Work out the finished part from the listing and answer in its coordinate system (mm). A direction names the side the tool comes from. Round coordinates to 2 decimals unless told otherwise and drop trailing zeros. Order: outer loops, then holes, each group sorted by start corner. A loop starts at its lowest first (then second) coordinate and runs counter-clockwise, first axis right, second up. Notation, with made-up numbers: M -14.5,38 L 14.5,38 A6 cw 14.5,45 Z; hole C 73,19 d8. An arc over 180 degrees is marked long. Return JSON: item names as keys, results as strings.
from build123d import *

# Parameters (mm, degrees)
SKETCH2_W           = 508
SKETCH2_H           = 101.6
BOSS_EXTRUDE2_DEPTH = 965.2
SKETCH3_R           = 25.4
SKETCH3_W           = 25.4
SKETCH3_H           = 25.4
CUT_EXTRUDE1_DEPTH  = 50.8
FILLET1_R           = 203.2
FILLET2_R           = 203.2
FILLET4_R           = 43.18


with BuildPart() as part:
    # Sketch2 → Boss-Extrude2 (new body)
    with BuildSketch(Plane.XY):
        with Locations((254, 50.8)):
            Rectangle(SKETCH2_W, SKETCH2_H)
    extrude(amount=BOSS_EXTRUDE2_DEPTH)

    # Sketch3 → Cut-Extrude1 (cut)
    with BuildSketch(Plane(origin=(0, 0, 0), x_dir=(-1, 0, 0), z_dir=(0, -1, 0))):
        with Locations(Location((-88.9, -736.6, 0), (0, 0, 90))):
            Circle(SKETCH3_R)
        with Locations(Location((-419.1, -736.6, 0), (0, 0, 90))):
            Circle(SKETCH3_R)
        with Locations((-393.7, -228.6)):
            Rectangle(SKETCH3_W, SKETCH3_H)
        with Locations((-114.3, -228.6)):
            Rectangle(SKETCH3_W, SKETCH3_H)
    extrude(amount=-CUT_EXTRUDE1_DEPTH, mode=Mode.SUBTRACT)

    # Fillet1
    fillet1_edges = [part.edges().sort_by_distance(p)[0] for p in [
        (0, 50.8, 965.2),
    ]]
    fillet(fillet1_edges, radius=FILLET1_R)

    # Fillet2
    fillet2_edges = [part.edges().sort_by_distance(p)[0] for p in [
        (508, 50.8, 965.2),
    ]]
    fillet(fillet2_edges, radius=FILLET2_R)

    # Fillet4
    fillet4_edges = [part.edges().sort_by_distance(p)[0] for p in [
        (254, 101.6, 965.2),
        (0, 101.6, 381),
        (59.515902063, 101.6, 905.684097937),
        (508, 101.6, 381),
        (254, 101.6, 0),
        (448.484097937, 101.6, 905.684097937),
    ]]
    fillet(fillet4_edges, radius=FILLET4_R)


solid = part.part
Item 1: Which of the six approach directions +Z, -Z, +X, -X, +Y, -Y give full straight-line access (tool end or side, diameter ignored) to faces 4 (the flat face through (251, 101.6, 476)), 5 (the flat face through (101.6, 25, 229))?
Output:
{"face 4": "+Z, -Z, +X, -X, +Y", "face 5": "-Y"}
Item 2: Find section B-B (z = 736.6). Determine the outline of the cut face in (x, y).
Output:
{"outline": "M 0,0 L 63.5,0 L 63.5,50.8 L 114.3,50.8 L 114.3,0 L 393.7,0 L 393.7,50.8 L 444.5,50.8 L 444.5,0 L 508,0 L 508,58.42 A43.18 ccw 464.82,101.6 L 43.18,101.6 A43.18 ccw 0,58.42 Z"}
Item 3: Consider line 1 along X through (y, z) = (18.5, 736.6); line 2 along Y through (x, z) = (398, 227.5); line 3 along Y through (x, z) = (467.5, 134.5). Determine where each line is inside the solid, lowest interval first. Write a range as [from, to].
Output:
{"line 1": "x = [0, 63.5], [114.3, 393.7], [444.5, 508]", "line 2": "y = [50.8, 101.6]", "line 3": "y = [0, 101.52]"}
Item 4: Find section C-C (z = 60.5). Determine the outline of the cut face in (x, y).
Output:
{"outline": "M 0,0 L 508,0 L 508,58.42 A43.18 ccw 464.82,101.6 L 43.18,101.6 A43.18 ccw 0,58.42 Z"}
Item 5: Each of these flat-tipped pins is pushed along its axis until it touches: pin 1 (12.5 mm diameter, centred on x = 391.5, y = 21, fed in from +Z); pin 2 (2 mm diameter, centred on y = 62.5, z = 480.5, fed in from -X); pin 3 (1.5 mm diameter, centred on y = 37, z = 856, fed in from -X). Where does it stop, or does it pass through?
Output:
{"pin 1": "stops at z = 948.6", "pin 2": "stops at x = 0.11", "pin 3": "stops at x = 22.66"}
Item 6: Find section A-A (y = 14.5). Determine the outline of the cut face in (x, z).
Output:
{"outline": "M 0,0 L 508,0 L 508,762 A203.2 ccw 304.8,965.2 L 203.2,965.2 A203.2 ccw 0,762 Z; hole C 88.9,736.6 d50.8; hole M 101.6,215.9 L 127,215.9 L 127,241.3 L 101.6,241.3 Z; hole M 381,215.9 L 406.4,215.9 L 406.4,241.3 L 381,241.3 Z; hole C 419.1,736.6 d50.8"}
Item 7: The mould has two halves that part along Z. Classify faces 1 (the cylindrical face through (446.896, 29.619, 907.255)), 2 (the flat face through (250, 0, 476)), 3 (the flat face through (394, 50.8, 228)): pulls with the +Z half, pulls with the -Z half, needs draft (parallel to the pull), parting line crosses it, or undercut.
Output:
{"face 1": "pulls with the +Z half", "face 2": "needs draft", "face 3": "undercut"}
